Answer from the drawing. Dimensions are ordinates in mm from the lowest x, y and z of the part. Give positions to 0.01 mm unless a question says otherwise; leave off trailing zeros. Write each loop counter-clockwise with the first axis right and the second up, starting at its lowest first coordinate (ties: lowest second). Pieces come first, ordered by that corner, then holes. Notation, with made-up numbers: M -4.5,54 L 42.5,54 A23 ccw 42.5,91 Z; hole C 55.25,16 d6. An arc over 180 degrees is marked long. Put each result on its own line as item: value.
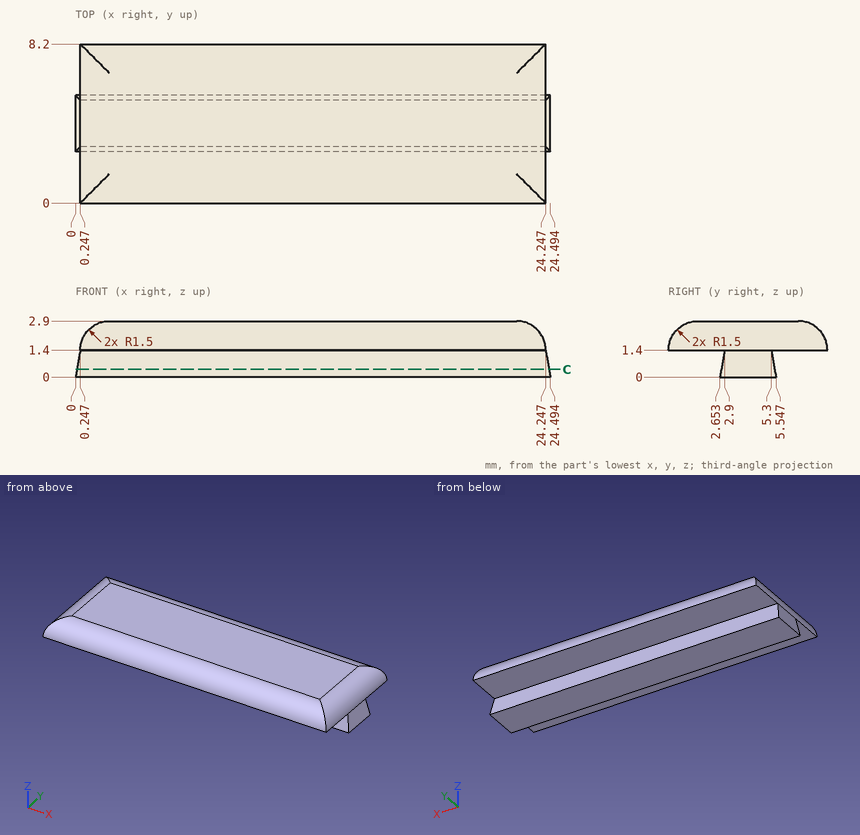
(1) Section C-C on z = 0.4 is taken. Determine the outline of the cut face in (x, y).
Result:
outline: M 0.07,2.72 L 24.42,2.72 L 24.42,5.48 L 0.07,5.48 Z
(2) Straight lines are drawn through the part: line 1 along Z through (x, y) = (17.5, 5.75); line 2 along Y through (x, z) = (14.75, 2.1); line 3 along Y through (x, z) = (14.5, 0.5). For each, find the intervals that lie inside material, in ascending order. Write a range as from..to.
Result:
line 1: z = 1.4..2.9
line 2: y = 0.17..8.03
line 3: y = 2.74..5.46
(3) Given pin 1 Ø3 at (x, y) = (14, 6.5) entering from -Z, flat-ended and moving along its own axis, determine where the tip first touches the part or whether it passes through.
Result:
pin 1: stops at z = 0
